Part print with two shaded views. Sizes in mm from the minimum x, y, z corner. Give positions to 0.01 mm unless a question says otherwise; leave off trailing zeros. Write each loop counter-clockwise with the first axis right and the second up, starting at its lowest first coordinate (ties: lowest second). Pieces come first, ordered by that corner, then holes. Notation, with made-up numbers: M 58,33.5 L 63,33.5 A24 ccw 63,56.5 Z; hole C 12.25,-19.5 d4. An arc over 180 degrees is marked long. Return JSON: item names as keys, results as strings. Group by question number.
Q1. Wall check: probe 1 along X at (y, z) = (84, 0.5) (1 decimal); probe 2 along X at (y, z) = (18.5, 1.05); probe 3 along Y at (x, z) = (19, 1.8) (1 decimal). Give the ranges that are in metal, low to high.
Q2. Flat gauge pin, fed straight in: pin 1 Ø2 at (x, y) = (49.95, 57.26) entering from -Z. Where does the tip first touch, or does it go through?
Q3. Band-saw the part on B-B, the plane y = 18.3. Give the cut face in (x, z) (1 decimal).
Q4. Band-saw the part on A-A, the plane y = 42.86. Give the cut face in (x, z) (1 decimal), then the cut area to 3 significant figures.
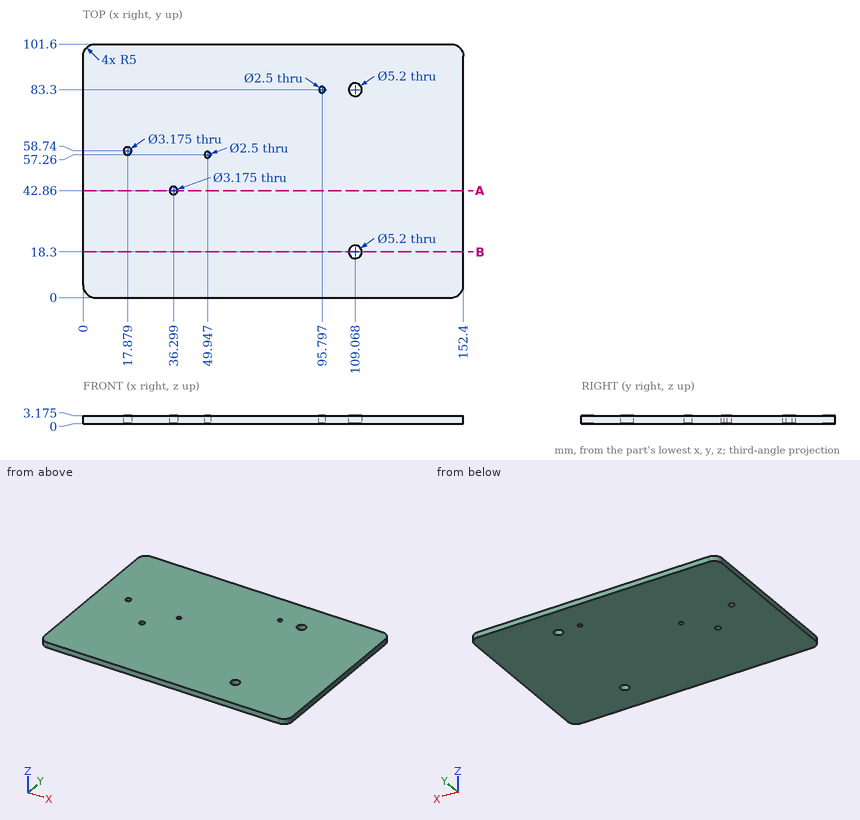
From the geometry:
{
 "1": {"probe 1": "x = 0 to 94.8, 96.8 to 106.6, 111.6 to 152.4", "probe 2": "x = 0 to 106.48, 111.66 to 152.4", "probe 3": "y = 0 to 57.6, 59.9 to 101.6"},
 "2": {"pin 1": "passes through"},
 "3": {"outline": "M 0,0 L 106.5,0 L 106.5,3.2 L 0,3.2 Z; M 111.7,0 L 152.4,0 L 152.4,3.2 L 111.7,3.2 Z"},
 "4": {"outline": "M 0,0 L 34.7,0 L 34.7,3.2 L 0,3.2 Z; M 37.9,0 L 152.4,0 L 152.4,3.2 L 37.9,3.2 Z", "area": "474 mm^2"}
}
